```python
from build123d import *

# Parameters (mm, degrees)
BOSS_EXTRUDE1_DEPTH     = 9.906
CUT_EXTRUDE1_DEPTH      = 18.304652958
CUT_EXTRUDE1_DEPTH_BACK = 7.493
SKETCH2_R               = 5.461
SKETCH2_R_2             = 3.683
SKETCH2_3_R             = 3.683
CUT_EXTRUDE2_DEPTH      = 18.304652958
SKETCH3_R               = 5.461
SKETCH3_R_2             = 3.683
CUT_EXTRUDE3_DEPTH      = 7.493
SKETCH3_4_R             = 3.683
CUT_EXTRUDE4_DEPTH      = 18.304652958


with BuildPart() as part:
    # Sketch1 → Boss-Extrude1 (new, symmetric)
    with BuildSketch(Plane(origin=(0, 0, 0), x_dir=(0, 0, -1), z_dir=(1, 0, 0))):
        Polygon((-10.033, -10.033), (10.033, 10.033), (10.033, -10.033), align=None)
    extrude(amount=BOSS_EXTRUDE1_DEPTH, both=True)

    # Sketch2 → Cut-Extrude1 (cut, two sides: drawn at the far end of the back side and taken through both)
    # profile 1 of 2: a face of its own
    with BuildSketch(Plane(origin=(0, 0, 0), x_dir=(1, 0, 0), z_dir=(0, 1, 0)).offset(-CUT_EXTRUDE1_DEPTH_BACK)):
        with Locations(Location((0, 0, 0), (0, 0, 270))):
            Circle(SKETCH2_R)
        Circle(SKETCH2_R_2, mode=Mode.SUBTRACT)
    # profile 2 of 2: a face of its own
    with BuildSketch(Plane(origin=(0, 0, 0), x_dir=(1, 0, 0), z_dir=(0, 1, 0)).offset(-CUT_EXTRUDE1_DEPTH_BACK)):
        Circle(SKETCH2_R_2)
    extrude(amount=CUT_EXTRUDE1_DEPTH + CUT_EXTRUDE1_DEPTH_BACK, mode=Mode.SUBTRACT)

    # Sketch2<3> → Cut-Extrude2 (cut, through all)
    with BuildSketch(Plane(origin=(0, 0, 0), x_dir=(1, 0, 0), z_dir=(0, 1, 0))):
        with Locations(Location((0, 0, 0), (0, 0, 270))):
            Circle(SKETCH2_3_R)
    extrude(amount=-CUT_EXTRUDE2_DEPTH, mode=Mode.SUBTRACT)

    # Sketch3 → Cut-Extrude3 (cut)
    # profile 1 of 2: a face of its own
    with BuildSketch(Plane.XY):
        Circle(SKETCH3_R)
        Circle(SKETCH3_R_2, mode=Mode.SUBTRACT)
    # profile 2 of 2: a face of its own
    with BuildSketch(Plane.XY):
        Circle(SKETCH3_R_2)
    extrude(amount=-CUT_EXTRUDE3_DEPTH, mode=Mode.SUBTRACT)

    # Sketch3<4> → Cut-Extrude4 (cut, through all)
    with BuildSketch(Plane.XY):
        Circle(SKETCH3_4_R)
    extrude(amount=-CUT_EXTRUDE4_DEPTH, mode=Mode.SUBTRACT)


solid = part.part
```
Can you work these out from the model? Positions are in its coordinate system, mm. A direction names the side the tool comes from. Give positions to 0.01 mm unless a question says otherwise; leave off trailing zeros. Loops run counter-clockwise (first coordinate to the right, second up) from the corner with the lowest first, then second, coordinate; pieces in that order, holes last. Notation, with made-up numbers: M -38,70 L -2,70 A19 cw -2,104 Z; hole C -18,19 d11. An arc over 180 degrees is marked long. One line per question, with ' | ' between items. Start each with the question number.
Q1. If we section it at B-B (y = -2.5): Please give me the cut outline in (x, z).
Q2. If we section it at A-A (x = 0): Please give me the cut outline in (y, z), plus the area to 3 significant figures.
Q3. For faces 4 (the flat face through (-9.906, -4, -5)), 5 (the flat face through (-4, -7.493, 1)), 6 (the cylindrical face through (-5.456, 0.24, -5.359)), which set-ups out of +Z, -Z, +X, -X, +Y, -Y let a thin tool reach every point of the face, with its end or its side?
Q4. For pin 1 Ø8.5 at (x, z) = (0, 0) entering from +Y; pin 2 Ø2 at (x, y) = (5, -3.5) entering from +Z; pin 3 Ø2 at (x, y) = (-7.5, -5) entering from +Z; pin 4 Ø2 at (y, z) = (-3.5, 5) entering from +X, each with a flat end and sliding along its axis, tell me the tip position at first contact or that it passes through.
Q5. If we section it at C-C (z = 3): Please give me the cut outline in (x, y).
Q6. If we section it at D-D (y = 1.5): Please give me the cut outline in (x, z), plus the area to 3 significant figures.
Q7. If we mould it in two halves opening along X, with no side actions, what happens to faces 1 (the flat face through (5, 0, -10.033)), 2 (the flat face through (9.906, -4, -5)), 3 (the flat face through (1, -4, -7.493))? For each: +X half, -X half, draft (parallel to the pull), parting line (faces both ways), or undercut.
Q8. If I drill on line 1 (X direction, y = -4.25, z = 0); line 2 (Z direction, x = 1.25, y = -4.5), over which ranges is the centre line in solid material (lowest first)? Write a range as from..to.
Computed:
1) outline: M -9.91,-10.03 L -2.7,-10.03 L -2.7,-7.49 L -4.86,-7.49 L -4.86,-2.5 A5.46 cw -4.86,2.5 L -9.91,2.5 Z; M 2.7,-10.03 L 9.91,-10.03 L 9.91,2.5 L 4.86,2.5 A5.46 cw 4.86,-2.5 L 4.86,-7.49 L 2.7,-7.49 Z
2) outline: M -10.03,-10.03 L -3.68,-10.03 L -3.68,-7.49 L -5.46,-7.49 L -5.46,-5.46 L -7.49,-5.46 L -7.49,-3.68 L -10.03,-3.68 Z; M -10.03,3.68 L -7.49,3.68 L -7.49,5.46 L -5.46,5.46 L -10.03,10.03 Z; M 3.68,-10.03 L 10.03,-10.03 L 5.46,-5.46 L 5.46,-7.49 L 3.68,-7.49 Z | area: 59.9 mm²
3) face 4: +Z, -Z, -X, +Y, -Y | face 5: +Y | face 6: +Z
4) pin 1: stops at y = -7.49 | pin 2: stops at z = 4.5 | pin 3: stops at z = 6 | pin 4: passes through
5) outline: M -9.91,-10.03 L -2.14,-10.03 L -2.14,-7.49 L -4.56,-7.49 L -4.56,-3 L -9.91,-3 Z; M 2.14,-10.03 L 9.91,-10.03 L 9.91,-3 L 4.56,-3 L 4.56,-7.49 L 2.14,-7.49 Z
6) outline: M -9.91,-10.03 L -3.36,-10.03 L -3.36,-7.49 L -5.25,-7.49 L -5.25,-1.5 L -9.91,-1.5 Z; M 3.36,-10.03 L 9.91,-10.03 L 9.91,-1.5 L 5.25,-1.5 L 5.25,-7.49 L 3.36,-7.49 Z | area: 89.0 mm²
7) face 1: draft | face 2: +X half | face 3: undercut
8) line 1: x = -9.91..-5.46, 5.46..9.91 | line 2: z = -10.03..-7.49
